from build123d import *

# Parameters (mm, degrees)
SKETCH_1_R          = 25.4
SKETCH_1_R_2        = 4
EXTRUDE_1_DEPTH     = 2
CUT_EXTRUDE_1_DEPTH = 36.9766591
SKETCH_3_R          = 1.25
SKETCH_3_R_2        = 5
CUT_EXTRUDE_2_DEPTH = 36.269108296
FILLET_1_R          = 0.5
SKETCH_4_R          = 1.55
CUT_EXTRUDE_3_DEPTH = 36.119904794
SKETCH_5_W          = 18.2
SKETCH_5_H          = 2
CUT_EXTRUDE_4_DEPTH = 2


with BuildPart() as part:
    # 草图1 → 凸台-拉伸1 (new body)
    with BuildSketch(Plane(origin=(0, 0, 0), x_dir=(1, 0, 0), z_dir=(0, 1, 0))):
        with Locations(Location((0, 0, 0), (0, 0, 270))):
            Circle(SKETCH_1_R)
        with Locations(Location((0, 0, 0), (0, 0, 270))):
            Circle(SKETCH_1_R_2, mode=Mode.SUBTRACT)
    extrude(amount=EXTRUDE_1_DEPTH)

    # 草图2 → 切除-拉伸1 (cut, through all)
    with BuildSketch(Plane(origin=(0, 2, 0), x_dir=(1, 0, 0), z_dir=(0, 1, 0))):
        with BuildLine():
            Line((-7.1, 24.387496797), (-7.1, 14.762503203))
            ThreePointArc((-7.1, 14.762503203), (0, 13.75), (7.1, 14.762503203))
            Line((7.1, 14.762503203), (7.1, 24.387496797))
            ThreePointArc((7.1, 24.387496797), (0, 25.4), (-7.1, 24.387496797))
        make_face()
        with BuildLine():
            Line((17.57019176, 18.342528765), (9.234702798, 13.530031969))
            ThreePointArc((9.234702798, 13.530031969), (11.907849302, 6.875), (16.334702798, 1.232471235))
            Line((16.334702798, 1.232471235), (24.67019176, 6.044968031))
            ThreePointArc((24.67019176, 6.044968031), (21.997045256, 12.7), (17.57019176, 18.342528765))
        make_face()
        with BuildLine():
            Line((24.67019176, -6.044968031), (16.334702798, -1.232471235))
            ThreePointArc((16.334702798, -1.232471235), (11.907849302, -6.875), (9.234702798, -13.530031969))
            Line((9.234702798, -13.530031969), (17.57019176, -18.342528765))
            ThreePointArc((17.57019176, -18.342528765), (21.997045256, -12.7), (24.67019176, -6.044968031))
        make_face()
        with BuildLine():
            Line((7.1, -24.387496797), (7.1, -14.762503203))
            ThreePointArc((7.1, -14.762503203), (0, -13.75), (-7.1, -14.762503203))
            Line((-7.1, -14.762503203), (-7.1, -24.387496797))
            ThreePointArc((-7.1, -24.387496797), (0, -25.4), (7.1, -24.387496797))
        make_face()
        with BuildLine():
            Line((-17.57019176, -18.342528765), (-9.234702798, -13.530031969))
            ThreePointArc((-9.234702798, -13.530031969), (-11.907849302, -6.875), (-16.334702798, -1.232471235))
            Line((-16.334702798, -1.232471235), (-24.67019176, -6.044968031))
            ThreePointArc((-24.67019176, -6.044968031), (-21.997045256, -12.7), (-17.57019176, -18.342528765))
        make_face()
        with BuildLine():
            Line((-24.67019176, 6.044968031), (-16.334702798, 1.232471235))
            ThreePointArc((-16.334702798, 1.232471235), (-11.907849302, 6.875), (-9.234702798, 13.530031969))
            Line((-9.234702798, 13.530031969), (-17.57019176, 18.342528765))
            ThreePointArc((-17.57019176, 18.342528765), (-21.997045256, 12.7), (-24.67019176, 6.044968031))
        make_face()
    extrude(amount=-CUT_EXTRUDE_1_DEPTH, mode=Mode.SUBTRACT)

    # 草图3 → 切除-拉伸2 (cut, through all)
    with BuildSketch(Plane(origin=(0, 2, 0), x_dir=(1, 0, 0), z_dir=(0, 1, 0))):
        with Locations(Location((-10.25, 17.753520778, 0), (0, 0, 270))):
            Circle(SKETCH_3_R)
        with Locations(Location((10.25, 17.753520778, 0), (0, 0, 270))):
            Circle(SKETCH_3_R)
        with Locations(Location((20.5, 0, 0), (0, 0, 270))):
            Circle(SKETCH_3_R)
        with Locations(Location((10.25, -17.753520778, 0), (0, 0, 270))):
            Circle(SKETCH_3_R)
        with Locations(Location((-10.25, -17.753520778, 0), (0, 0, 270))):
            Circle(SKETCH_3_R)
        with Locations(Location((-20.5, 0, 0), (0, 0, 270))):
            Circle(SKETCH_3_R)
        with Locations((-29, 0)):
            Circle(SKETCH_3_R_2)
        with Locations((-14.5, 25.11473671)):
            Circle(SKETCH_3_R_2)
        with Locations((14.5, 25.11473671)):
            Circle(SKETCH_3_R_2)
        with Locations((29, 0)):
            Circle(SKETCH_3_R_2)
        with Locations((14.5, -25.11473671)):
            Circle(SKETCH_3_R_2)
        with Locations((-14.5, -25.11473671)):
            Circle(SKETCH_3_R_2)
    extrude(amount=-CUT_EXTRUDE_2_DEPTH, mode=Mode.SUBTRACT)

    # 圆角1
    fillet_1_edges = [part.edges().sort_by_distance(p)[0] for p in [
        (16.334702798, 1, -1.232471235),
        (9.234702798, 1, -13.530031969),
        (9.234702798, 1, 13.530031969),
        (16.334702798, 1, 1.232471235),
        (-7.1, 1, 14.762503203),
        (7.1, 1, 14.762503203),
        (-9.234702798, 1, 13.530031969),
        (-9.234702798, 1, -13.530031969),
        (-16.334702798, 1, -1.232471235),
        (7.1, 1, -14.762503203),
        (-7.1, 1, -14.762503203),
    ]]
    fillet(fillet_1_edges, radius=FILLET_1_R)

    # 草图4 → 切除-拉伸3 (cut, through all)
    with BuildSketch(Plane(origin=(0, 2, 0), x_dir=(1, 0, 0), z_dir=(0, 1, 0))):
        with Locations(Location((-7, 0, 0), (0, 0, 270))):
            Circle(SKETCH_4_R)
        with Locations(Location((0, 7, 0), (0, 0, 270))):
            Circle(SKETCH_4_R)
        with Locations(Location((7, 0, 0), (0, 0, 270))):
            Circle(SKETCH_4_R)
        with Locations(Location((0, -7, 0), (0, 0, 270))):
            Circle(SKETCH_4_R)
    extrude(amount=-CUT_EXTRUDE_3_DEPTH, mode=Mode.SUBTRACT)

    # 草图5 → 切除-拉伸4 (cut)
    with BuildSketch(Plane(origin=(0, 2, 0), x_dir=(1, 0, 0), z_dir=(0, 1, 0))):
        Polygon((-12.337495374, -17.630831174), (-21.437495374, -1.869168826), (-23.169546181, -2.869168826), (-14.069546181, -18.630831174), align=None)
        Polygon((-14.069546181, 18.630831174), (-12.337495374, 17.630831174), (-21.437495374, 1.869168826), (-23.169546181, 2.869168826), align=None)
        with Locations((0, 20.5)):
            Rectangle(SKETCH_5_W, SKETCH_5_H)
        Polygon((23.169546181, 2.869168826), (21.437495374, 1.869168826), (12.337495374, 17.630831174), (14.069546181, 18.630831174), align=None)
        Polygon((14.069546181, -18.630831174), (12.337495374, -17.630831174), (21.437495374, -1.869168826), (23.169546181, -2.869168826), align=None)
        with Locations((0, -20.5)):
            Rectangle(SKETCH_5_W, SKETCH_5_H)
    extrude(amount=-CUT_EXTRUDE_4_DEPTH, mode=Mode.SUBTRACT)


solid = part.part
CAD build for the part. Positions are in the model's coordinates, mm. A direction names the side the tool comes from. Round coordinates to 2 decimals unless told otherwise and drop trailing zeros. Write each loop counter-clockwise with the first axis right and the second up, starting at its lowest first coordinate (ties: lowest second). Pieces come first, ordered by that corner, then holes. Notation, with made-up numbers: M 24,56.5 L 78,56.5 A17 ccw 78,62.5 Z; hole C -7,75 d4. An arc over 180 degrees is marked long. Put each result on its own line as item: value. Start each with the question number.
1) Saw through at A-A, the plane z = 0. Write the cut outline in (x, y), and give its area (3 significant figures).
2) Drill centre lines: probe 1 along X at (y, z) = (0.7, 0); probe 2 along Z at (x, y) = (-17, 1.7); probe 3 along X at (y, z) = (1, -5). Where is each one in solid material? Low to high. Write a range as [from, to].
3) Pin check, flat tips, straight feed: pin 1 Ø3 at (x, z) = (20.5, 0) entering from +Y; pin 2 Ø1 at (x, y) = (-8, 1) entering from -Z; pin 3 Ø0.6 at (x, y) = (8, 1) entering from -Z; pin 4 Ø1 at (y, z) = (1, -18) entering from -X. Stop position of each tip, or through.
4) Saw through at C-C, the plane y = 0.4. Count the separate pieces of the cut face and the enclosed holes in it, and give its area (3 significant figures).
5) 3-axis set-ups, long thin cutter, end or side, ignore diameter. For faces 5 (the flat face through (7.1, 1, -17)), 6 (the cylindrical face through (-24.967, 0.986, -4.67)), 7 (the flat face through (8, 1, -21.5)): which of +Z, -Z, +X, -X, +Y, -Y reach the whole face in a straight line?
6) Saw through at B-B, the plane z = 7. Write the cut outline in (x, y), and give its area (3 significant figures).
7) Pull direction X, two halves, no side cores. Call faces 1 (the cylindrical face through (-10.195, 1.014, 16.505)), 2 (the cylindrical face through (8.477, 0.986, -23.944)), 3 (the flat face through (-16.3, 1.01, -17.61)), 4 (the cylindrical face through (-12.04, 1.01, -20.76)): pulls with the +X half, pulls with the -X half, needs draft (parallel to the pull), parting line crosses it, or undercut.
Resolved:
1. outline: M -24,0 L -21.75,0 L -21.75,2 L -24,2 Z; M -19.25,0 L -8.55,0 L -8.55,2 L -19.25,2 Z; M -5.45,0 L -4,0 L -4,2 L -5.45,2 Z; M 4,0 L 5.45,0 L 5.45,2 L 4,2 Z; M 8.55,0 L 19.25,0 L 19.25,2 L 8.55,2 Z; M 21.75,0 L 24,0 L 24,2 L 21.75,2 Z
1. area: 57.6 mm²
2. probe 1: [-24, -21.75], [-19.25, -8.55], [-5.45, -4], [4, 5.45], [8.55, 19.25], [21.75, 24]
2. probe 2: [-18.87, -18.01], [-1.62, 1.62], [18.01, 18.87]
2. probe 3: [-24.9, -22.86], [-13.1, 13.1], [22.86, 24.9]
3. pin 1: y = 2
3. pin 2: z = -24.27
3. pin 3: z = -24.2
3. pin 4: x = -17.57
4. separate pieces: 1
4. enclosed holes: 11
4. area: 897 mm²
5. face 5: -Z, +Y, -Y
5. face 6: -Z, -X, +Y, -Y
5. face 7: +Y, -Y
6. outline: M -11.84,0 L -1.55,0 L -1.55,2 L -11.84,2 Z; M 1.55,0 L 11.84,0 L 11.84,2 L 1.55,2 Z
6. area: 41.1 mm²
7. face 1: undercut
7. face 2: pulls with the +X half
7. face 3: pulls with the -X half
7. face 4: undercut
